CAD build for the part. Positions are in the model's coordinates, mm. A direction names the side the tool comes from. Round coordinates to 2 decimals unless told otherwise and drop trailing zeros. Order: outer loops, then holes, each group sorted by start corner. A loop starts at its lowest first (then second) coordinate and runs counter-clockwise, first axis right, second up. Notation, with made-up numbers: (-16.5, 28) - (24.5, 28) arc R9 cw to (24.5, 39) - close; hole circle Ø5 at (68, -20.75). An arc over 180 degrees is marked (long way). Write item = value, one per line.
from build123d import *

# Parameters (mm, degrees)
F0_R      = 50
F1_DEPTH  = 4
F2_R      = 25
F3_DEPTH  = 40
F5_DEPTH  = 5.8
F6_DEPTH  = 5.8
F7_DEPTH  = 5.8
F8_R      = 45
F9_DEPTH  = 4
F10_W     = 6
F10_H     = 6
F11_DEPTH = 4
F12_R     = 25
F13_DEPTH = 5
F14_R     = 22.5
F15_DEPTH = 40


with BuildPart() as f1:
    # F0 (on Top) → F1 (new body)
    with BuildSketch(Plane.XY):
        Circle(F0_R)
    extrude(amount=F1_DEPTH)

    # F2 (on face) → F3 (join)
    with BuildSketch(Plane.XY.offset(4)):
        Circle(F2_R)
    extrude(amount=F3_DEPTH)

    # F4 (on face) → F5 (join)
    with BuildSketch(Plane.XY.offset(4)):
        with BuildLine():
            ThreePointArc((5, 49.7493718553), (2.503138753, 49.9373036555), (0, 50))
            ThreePointArc((0, 50), (-2.503138753, 49.9373036555), (-5, 49.7493718553))
            Line((-5, 49.7493718553), (-5, 44.5003296036))
            Line((-5, 44.5003296036), (5, 44.5003296036))
            Line((5, 44.5003296036), (5, 49.7493718553))
        make_face()
    extrude(amount=F5_DEPTH)

    # F4 (on face) → F6 (join)
    with BuildSketch(Plane.XY.offset(4)):
        with BuildLine():
            ThreePointArc((0, -50), (2.503138753, -49.9373036555), (5, -49.7493718553))
            Line((5, -49.7493718553), (5, -44))
            Line((5, -44), (-5, -44))
            Line((-5, -44), (-5, -49.7493718553))
            ThreePointArc((-5, -49.7493718553), (-2.503138753, -49.9373036555), (0, -50))
        make_face()
    extrude(amount=F6_DEPTH)

    # F4 (on face) → F7 (join)
    with BuildSketch(Plane.XY.offset(4)):
        with BuildLine():
            Line((-44, 5), (-49.7493718553, 5))
            ThreePointArc((-49.7493718553, 5), (-49.9373036555, 2.503138753), (-50, 0))
            ThreePointArc((-50, 0), (-49.9373036555, -2.503138753), (-49.7493718553, -5))
            Line((-49.7493718553, -5), (-44, -5))
            Line((-44, -5), (-44, 5))
        make_face()
        with BuildLine():
            ThreePointArc((50, 0), (49.9373036555, 2.503138753), (49.7493718553, 5))
            Line((49.7493718553, 5), (44, 5))
            Line((44, 5), (44, -5))
            Line((44, -5), (49.7493718553, -5))
            ThreePointArc((49.7493718553, -5), (49.9373036555, -2.503138753), (50, 0))
        make_face()
    extrude(amount=F7_DEPTH)

    # F8 (on Top) → F9 (cut)
    with BuildSketch(Plane.XY):
        Circle(F8_R)
    extrude(amount=F9_DEPTH, mode=Mode.SUBTRACT)

    # F10 (on Top) → F11 (join)
    with BuildSketch(Plane.XY):
        Polygon((6, 46.8811020255), (-6, 46.8811020255), (-6, 6), (0, 6), (6, 6), align=None)
        with Locations((-3, 3)):
            Rectangle(F10_W, F10_H)
        Polygon((-6, 0), (-6, 6), (-46.5700030327, 6), (-46.5700030327, -6), (-6, -6), align=None)
        Polygon((46.8255914748, 6), (6, 6), (6, 0), (6, -6), (46.8255914748, -6), align=None)
        with Locations((3, 3)):
            Rectangle(F10_W, F10_H)
        with Locations((-3, -3)):
            Rectangle(F10_W, F10_H)
        with Locations((3, -3)):
            Rectangle(F10_W, F10_H)
        Polygon((0, -6), (-6, -6), (-6, -46.7753745615), (6, -46.7753745615), (6, -6), align=None)
    extrude(amount=F11_DEPTH)

    # F12 (on Top) → F13 (join)
    with BuildSketch(Plane.XY):
        Circle(F12_R)
    extrude(amount=F13_DEPTH)

    # F14 (on face) → F15 (cut)
    with BuildSketch(Plane(origin=(0, 0, 0), x_dir=(1, 0, 0), z_dir=(0, 0, -1))):
        Circle(F14_R)
    extrude(amount=-F15_DEPTH, mode=Mode.SUBTRACT)


solid = f1.part
(1) Band-saw the part on C-C on x = 36. List the corners of the cut face in (y, z), plus the area to 3 significant figures.
Solved:
outline = (-34.7, 0) - (-27, 0) - (-27, 4) - (-34.7, 4) - close; (-6, 0) - (6, 0) - (6, 4) - (-6, 4) - close; (27, 0) - (34.7, 0) - (34.7, 4) - (27, 4) - close
area = 110 mm²
(2) Tool access for faces 4 (the flat face through (5, -47, 7)), 5 (the flat face through (-5, 47, 7)), 6 (the flat face through (-6, -34, 2)), 7 (the cylindrical face through (10.382, 19.961, 19.72)), 8 (the flat face through (0, -47, 9.8)): list every direction of +Z, -Z, +X, -X, +Y, -Y with a clear straight run to the whole face (end or side of a thin tool).
Solved:
face_4 = +Z, +X, -Y
face_5 = +Z, -X, +Y
face_6 = +Z, -Z
face_7 = -Z
face_8 = +Z, +X, -X, -Y
(3) Pull direction Y, two halves, no side cores. Call faces 1 (the flat face through (-35, -6, 2)), 2 (the flat face through (-22.5, 3.9, 0)), 3 (the flat face through (47, 5, 7)): released by +Y, released by -Y, zero draft, split by the parting line, or undercut.
Solved:
face_1 = undercut
face_2 = zero draft
face_3 = released by +Y
(4) Band-saw the part on D-D on x = -3. List the corners of the cut face in (y, z).
Solved:
outline = (-49.91, 0) - (-22.3, 0) - (-22.3, 40) - (22.3, 40) - (22.3, 0) - (49.91, 0) - (49.91, 9.8) - (44.5, 9.8) - (44.5, 4) - (24.82, 4) - (24.82, 44) - (-24.82, 44) - (-24.82, 4) - (-44, 4) - (-44, 9.8) - (-49.91, 9.8) - close
(5) Drop flat-ended pins along their axis: pin 1 (3 mm diameter, centred on x = -1, z = 7.5, fed in from +Y); pin 2 (5 mm diameter, centred on x = -10.5, y = 33, fed in from -Z); pin 3 (1 mm diameter, centred on x = -8, z = 6, fed in from +Y); pin 4 (6.5 mm diameter, centred on x = 47, y = 2, fed in from +Z). Give the stop position or say it passes through.
Solved:
pin_1 = 50
pin_2 = through
pin_3 = 23.85
pin_4 = 9.8
(6) Band-saw the part on B-B on z = 36. List the corners of the cut face in (x, y), plus the area to 3 significant figures.
Solved:
outline = circle Ø50 at (0, 0); hole circle Ø45 at (0, 0)
area = 373 mm²
(7) Band-saw the part on A-A on y = 39. List the corners of the cut face in (x, z).
Solved:
outline = (-31.29, 0) - (-22.45, 0) - (-22.45, 4) - (-31.29, 4) - close; (-6, 0) - (6, 0) - (6, 4) - (-6, 4) - close; (22.45, 0) - (31.29, 0) - (31.29, 4) - (22.45, 4) - close
(8) Probe line 1 along X through (y, z) = (0, 30); line 2 along Y through (x, z) = (2, 23). List the from-to ranges inside material, lowest first.
Solved:
line_1 = -25 to -22.5, 22.5 to 25
line_2 = -24.92 to -22.41, 22.41 to 24.92
